Autodesk Inventor part; units mm, degrees
sketch "Sketch1" plane through (0, 0, 0) normal (0, 0, 1) x (1, 0, 0)
  line L0 (0, 0) -> (4, 0)
  line L1 (0, 0) -> (-4, 0)
  line L2 (-4, 7) -> (-4, 9.5)
  line L3 (4, 7) -> (4, 9.5)
  line L4 (-4, 7) -> (-8, 7)
  line L5 (4, 7) -> (8, 7)
  line L6 (-8, 7) -> (-8, 5)
  line L7 (8, 7) -> (8, 5)
  line L8 (8, 5) -> (4, 0)
  line L9 (-8, 5) -> (-4, 0)
  line L10 (-4, 9.5) -> (-15, 9.5)
  line L11 (4, 9.5) -> (15, 9.5)
  line L12 (-15, 9.5) -> (-15, 13.5)
  line L13 (-15, 13.5) -> (15, 13.5)
  line L14 (15, 13.5) -> (15, 9.5)
  dimension "d12" = 4
extrude "Extrusion1" add sketch "Sketch1" along normal blind 30
sketch "Sketch2" plane through (-15, 13.5, 0) normal (0, 1, 0) x (1, 0, 0)
  line L0 (0, -30) -> (11, -30)
  line L1 (30, 0) -> (30, -30)
  line L2 (30, 0) -> (0, 0)
  circle A0 centre (5, -5) radius 1.5
  circle A1 centre (5, -25) radius 1.5
  circle A2 centre (25, -25) radius 1.5
  circle A3 centre (25, -5) radius 1.5
  point P0 (15, 0)
  point P1 (15, -15)
  dimension "d19" = 360
extrude "Extrusion2" cut sketch "Sketch2" against normal blind 5
sketch "Sketch3" plane through (-15, 9.5, 0) normal (0, -1, 0) x (1, 0, 0)
  line L0 (3.5, 7.5981) -> (6.5, 7.5981)
  line L1 (6.5, 7.5981) -> (8, 5)
  line L2 (8, 5) -> (6.5, 2.4019)
  line L3 (6.5, 2.4019) -> (3.5, 2.4019)
  line L4 (3.5, 2.4019) -> (2, 5)
  line L5 (2, 5) -> (3.5, 7.5981)
  line L6 (3.5, 27.5981) -> (6.5, 27.5981)
  line L7 (6.5, 27.5981) -> (8, 25)
  line L8 (8, 25) -> (6.5, 22.4019)
  line L9 (6.5, 22.4019) -> (3.5, 22.4019)
  line L10 (3.5, 22.4019) -> (2, 25)
  line L11 (2, 25) -> (3.5, 27.5981)
  line L12 (23.5, 7.5981) -> (26.5, 7.5981)
  line L13 (26.5, 7.5981) -> (28, 5)
  line L14 (28, 5) -> (26.5, 2.4019)
  line L15 (26.5, 2.4019) -> (23.5, 2.4019)
  line L16 (23.5, 2.4019) -> (22, 5)
  line L17 (22, 5) -> (23.5, 7.5981)
  line L18 (23.5, 27.5981) -> (26.5, 27.5981)
  line L19 (26.5, 27.5981) -> (28, 25)
  line L20 (28, 25) -> (26.5, 22.4019)
  line L21 (26.5, 22.4019) -> (23.5, 22.4019)
  line L22 (23.5, 22.4019) -> (22, 25)
  line L23 (22, 25) -> (23.5, 27.5981)
  point P0 (15, 0)
  dimension "d23" = 3
  dimension "d24" = 3
  dimension "d26" = 3
  dimension "d27" = 120
  dimension "d28" = 3
  dimension "d29" = 120
  dimension "d30" = 3
  dimension "d31" = 3
  dimension "d32" = 120
  dimension "d33" = 3
  dimension "d34" = 120
  dimension "d35" = 3
  dimension "d36" = 120
  dimension "d37" = 3
  dimension "d38" = 3
  dimension "d40" = 3
  dimension "d41" = 120
  dimension "d42" = 3
  dimension "d43" = 120
  dimension "d44" = 3
  dimension "d45" = 3
  dimension "d46" = 120
  dimension "d47" = 3
  dimension "d48" = 120
  dimension "d49" = 3
  dimension "d50" = 120
extrude "Extrusion3" cut sketch "Sketch3" against normal blind 2.2
sketch "Sketch4" plane through (0, 0, 30) normal (0, 0, 1) x (1, 0, 0)
  line L0 (-8, 7) -> (-8, 5)
  line L1 (-8, 5) -> (-4, 0)
  line L2 (-4, 0) -> (4, 0)
  line L3 (4, 0) -> (8, 5)
  line L4 (8, 5) -> (8, 7)
  line L5 (8, 7) -> (4, 7)
  line L6 (4, 7) -> (4, 9.5)
  line L7 (4, 9.5) -> (15, 9.5)
  line L8 (15, 9.5) -> (15, 13.5)
  line L9 (15, 13.5) -> (-15, 13.5)
  line L10 (-15, 13.5) -> (-15, 9.5)
  line L11 (-15, 9.5) -> (-4, 9.5)
  line L12 (-4, 9.5) -> (-4, 7)
  line L13 (-4, 7) -> (-8, 7)
  line L14 (-8, 7) -> (-8, 5)
  line L15 (-8, 5) -> (-4, 0)
  line L16 (-4, 0) -> (4, 0)
  line L17 (4, 0) -> (8, 5)
  line L18 (8, 5) -> (8, 7)
  line L19 (8, 7) -> (4, 7)
  line L20 (4, 7) -> (4, 9.5)
  line L21 (4, 9.5) -> (15, 9.5)
  line L22 (15, 9.5) -> (15, 13.5)
  line L23 (15, 13.5) -> (-15, 13.5)
  line L24 (-15, 13.5) -> (-15, 9.5)
  line L25 (-15, 9.5) -> (-4, 9.5)
  line L26 (-4, 9.5) -> (-4, 7)
  line L27 (-4, 7) -> (-8, 7)
extrude "Extrusion4" add sketch "Sketch4" along normal blind 2
sketch "Sketch5" plane through (-15, 9.5, 0) normal (-1, 0, 0) x (0, 0, 1)
  line L0 (0, 4) -> (0, 0)
  line L1 (0, 0) -> (32, 0)
  line L2 (32, 4) -> (32, 0)
  line L3 (0, 4) -> (32, 4)
  point P0 (0, -9.5)
extrude "Extrusion5" add sketch "Sketch5" along normal blind 2
sketch "Sketch6" plane through (15, 9.5, 0) normal (1, 0, 0) x (0, 0, -1)
  line L0 (0, 0) -> (0, 4)
  line L1 (0, 4) -> (-32, 4)
  line L2 (-32, 0) -> (-32, 4)
  line L3 (0, 0) -> (-32, 0)
  point P0 (0, -9.5)
extrude "Extrusion6" add sketch "Sketch6" along normal blind 2
sketch "Sketch7" plane through (0, 0, 0) normal (0, 0, -1) x (-1, 0, 0)
  line L0 (8, 7) -> (8, 5)
  line L1 (4, 7) -> (8, 7)
  line L2 (4, 9.5) -> (4, 7)
  line L3 (4, 9.5) -> (17, 9.5)
  line L4 (17, 13.5) -> (17, 9.5)
  line L5 (17, 13.5) -> (-17, 13.5)
  line L6 (-17, 9.5) -> (-17, 13.5)
  line L7 (-4, 9.5) -> (-17, 9.5)
  line L8 (-4, 7) -> (-4, 9.5)
  line L9 (-8, 7) -> (-4, 7)
  line L10 (-8, 5) -> (-8, 7)
  line L11 (-4, 0) -> (-8, 5)
  line L12 (4, 0) -> (-4, 0)
  line L13 (8, 5) -> (4, 0)
  point P0 (0, 0)
extrude "Extrusion7" add sketch "Sketch7" along normal blind 2
sketch "Sketch8" plane through (0, 0, 32) normal (0, 0, 1) x (1, 0, 0)
  line L0 (-4, 7) -> (-8, 7)
  line L1 (-4, 7) -> (-4, 6.5)
  line L2 (-4, 6.5) -> (-8, 6.5)
  line L3 (-8, 7) -> (-8, 5)
  line L4 (-8, 7) -> (-4, 7)
  line L5 (3.9883, 6.9999) -> (3.9883, 6.4999)
  line L6 (3.9883, 6.4999) -> (8, 6.4999)
  line L7 (8, 5) -> (8, 7)
  line L8 (8, 6.4999) -> (8, 7)
  line L9 (8, 7) -> (4, 7)
  line L10 (8, 7) -> (4, 7)
  point P0 (0, 0)
  dimension "d61" = 0.5
extrude "Extrusion8" cut sketch "Sketch8" against normal blind 40
sketch "Sketch9" plane through (0, 0, 32) normal (0, 0, 1) x (1, 0, 0)
  line L0 (4, 7) -> (4, 9.5)
  line L1 (4, 7) -> (4, 6.5)
  line L2 (4, 6.5) -> (8, 6.5)
  line L3 (8, 7) -> (8, 5)
  line L4 (4, 7) -> (8, 7)
  line L5 (8, 7) -> (4, 7)
  point P0 (0, 0)
  dimension "d64" = 0.5
extrude "Extrusion9" cut sketch "Sketch9" against normal blind 40
sketch "Sketch10" plane through (-17, 9.5, 32) normal (0, -1, 0) x (1, 0, 0)
  line L0 (5.5, -24.4019) -> (8.5, -24.4019)
  line L1 (5.25, -30.0311) -> (3.5, -27)
  line L2 (5.25, -23.9689) -> (3.5, -27)
  line L3 (5.25, -23.9689) -> (8.75, -23.9689)
  line L4 (5.25, -30.0311) -> (8.75, -30.0311)
  line L5 (8.75, -30.0311) -> (10.5, -27)
  line L6 (10.5, -27) -> (8.75, -23.9689)
  line L7 (5.5, -9.5981) -> (4, -7)
  line L8 (30, -27) -> (28.5, -29.5981)
  line L9 (25.5, -4.4019) -> (28.5, -4.4019)
  line L10 (8.5, -9.5981) -> (5.5, -9.5981)
  line L11 (5.25, -10.0311) -> (3.5, -7)
  line L12 (5.25, -3.9689) -> (3.5, -7)
  line L13 (5.25, -3.9689) -> (8.75, -3.9689)
  line L14 (5.25, -10.0311) -> (8.75, -10.0311)
  line L15 (8.75, -10.0311) -> (10.5, -7)
  line L16 (10.5, -7) -> (8.75, -3.9689)
  line L17 (25.25, -10.0311) -> (23.5, -7)
  line L18 (25.25, -3.9689) -> (23.5, -7)
  line L19 (25.25, -3.9689) -> (28.75, -3.9689)
  line L20 (25.25, -10.0311) -> (28.75, -10.0311)
  line L21 (28.75, -10.0311) -> (30.5, -7)
  line L22 (30.5, -7) -> (28.75, -3.9689)
  line L23 (25.25, -30.0311) -> (23.5, -27)
  line L24 (25.25, -23.9689) -> (23.5, -27)
  line L25 (25.25, -23.9689) -> (28.75, -23.9689)
  line L26 (25.25, -30.0311) -> (28.75, -30.0311)
  line L27 (28.75, -30.0311) -> (30.5, -27)
  line L28 (30.5, -27) -> (28.75, -23.9689)
  point P0 (17, -32)
extrude "Extrusion10" cut sketch "Sketch10" against normal blind 2.2
properties part number "IDOM_infrared_fixture1"
Verification items for the finished model (mm, model axes). A direction names the side the tool comes from. Give positions to 0.01 mm unless a question says otherwise; leave off trailing zeros. Loops run counter-clockwise (first coordinate to the right, second up) from the corner with the lowest first, then second, coordinate; pieces in that order, holes last. Notation, with made-up numbers: (24.5, 80) - (83.5, 80) arc R6 cw to (83.5, 89) - close; hole circle Ø9 at (34, -36.5). An arc over 180 degrees is marked (long way). Write item = value, one per line. Start each with the question number.
Q1. Cross-section at D-D, the plane y = 8.5. Enter the section's corners in (x, z).
Q2. Cross-section at A-A, the plane x = -10. Enter the section's corners in (y, z).
Q3. Cross-section at B-B, the plane x = -5. Enter the section's corners in (y, z), and give its area (4 significant figures).
Q4. Cross-section at C-C, the plane z = 21.5. Enter the section's corners in (x, y), and give its area (3 significant figures).
Q5. Depth check by flat-ended pin: P1, Ø1.8, axis at x = 10, z = 24, coming from the -Y side; P2, Ø4, axis at y = 2.5, z = 3, coming from the +X side; P3, Ø3, axis at x = -9, z = 5, coming from the -Y side (3 decimals). Enter the tip coordinate at first touch or a pass-through.
Q6. Thickness scan on line 1 (Z direction, x = 10, y = 12.4); line 2 (X direction, y = 12.65, z = 25); line 3 (Y direction, x = 14, z = 6). Record the ranges inside material, lowest first.
Q7. Tool access check on faces 1 (the face through (12.61, 10.58, 23.46)), 2 (the face through (-7.39, 10.58, 3.46)), 3 (the face through (8, 6, 15)). Record the directions out of +Z, -Z, +X, -X, +Y, -Y that give a thin tool (end or side, any length) a straight path to the whole face; none if there is none.
Q8. Mould release check, pull along X, two halves, no side actions. Record for faces 4 (the face through (-12.61, 10.58, 6.54)), 5 (the face through (-17, 12, 15)), 6 (the face through (10, 9.5, 15)): released by +X, released by -X, zero draft, split by the parting line, or undercut.
Answer key:
q1.outline = (-4, -2) - (4, -2) - (4, 32) - (-4, 32) - close
q2.outline = (9.5, -2) - (13.5, -2) - (13.5, 3.5) - (11.7, 3.5) - (11.7, 1.97) - (9.5, 1.97) - close; (9.5, 8.03) - (11.7, 8.03) - (11.7, 6.5) - (13.5, 6.5) - (13.5, 23.5) - (11.7, 23.5) - (11.7, 21.97) - (9.5, 21.97) - close; (9.5, 28.03) - (11.7, 28.03) - (11.7, 26.5) - (13.5, 26.5) - (13.5, 32) - (9.5, 32) - close
q3.outline = (1.25, -2) - (6.5, -2) - (6.5, 32) - (1.25, 32) - close; (9.5, -2) - (13.5, -2) - (13.5, 32) - (9.5, 32) - close
q3.area = 314.5 mm^2
q4.outline = (-17, 9.5) - (-4, 9.5) - (-4, 6.5) - (-8, 6.5) - (-8, 5) - (-4, 0) - (4, 0) - (8, 5) - (8, 6.5) - (4, 6.5) - (4, 9.5) - (17, 9.5) - (17, 13.5) - (-17, 13.5) - close
q4.area = 244 mm^2
q5.P1 = 11.7
q5.P2 = 7.6
q5.P3 = 4.375
q6.line_1 = -2 to 3.5, 6.5 to 23.5, 26.5 to 32
q6.line_2 = -17 to -11.5, -8.5 to 8.5, 11.5 to 17
q6.line_3 = 9.5 to 13.5
q7.face_1 = -Y
q7.face_2 = none
q7.face_3 = +Z, -Z, +X, -Y
q8.face_4 = undercut
q8.face_5 = released by -X
q8.face_6 = zero draft
